Geometry check sheet. Reference: the model listing, model coordinates, mm. Round coordinates to 2 decimals unless told otherwise and drop trailing zeros. Write each loop counter-clockwise with the first axis right and the second up, starting at its lowest first coordinate (ties: lowest second). Pieces come first, ordered by that corner, then holes.
Item 1: Scan lines: probe 1 along Y at (x, z) = (589, 0); probe 2 along X at (y, z) = (-140, -45); probe 3 along Z at (x, y) = (953, 23). Record each from-to range of solid material in increasing order.
Item 2: Depth check by flat-ended pin: P1, Ø5, axis at x = 296, z = 9.5, coming from the -Y side; P2, Ø12, axis at x = 477, y = -91.5, coming from the -Z side; P3, Ø4, axis at x = 414, y = 117.5, coming from the +Z side. Enter the tip coordinate at first touch or a pass-through.
Item 3: Cross-section at C-C (x = 1178). Enter the section's corners in (y, z).
Item 4: Cross-section at A-A (y = 0). Enter the section's corners in (x, z).
from build123d import *

# Parameters (mm, degrees)
SKETCH1_R           = 158.75
SKETCH1_R_2         = 95.25
BOSS_EXTRUDE1_DEPTH = 1270
FILLET1_R           = 12.7
FILLET2_R           = 12.7


with BuildPart() as part:
    # Sketch1 → Boss-Extrude1 (new body)
    with BuildSketch(Plane(origin=(0, 0, 0), x_dir=(0, 0, -1), z_dir=(1, 0, 0))):
        Circle(SKETCH1_R)
        Circle(SKETCH1_R_2, mode=Mode.SUBTRACT)
    extrude(amount=BOSS_EXTRUDE1_DEPTH)

    # Fillet1
    fillet1_edges = [part.edges().sort_by_distance(p)[0] for p in [
        (1270, 0, 158.75),
        (1270, 0, 95.25),
    ]]
    fillet(fillet1_edges, radius=FILLET1_R)

    # Fillet2
    fillet2_edges = [part.edges().sort_by_distance(p)[0] for p in [
        (0, 0, 158.75),
        (0, 0, 95.25),
    ]]
    fillet(fillet2_edges, radius=FILLET2_R)


solid = part.part
Resolved:
1. probe 1: y = -158.75 to -95.25, 95.25 to 158.75
1. probe 2: x = 0.04 to 1269.96
1. probe 3: z = -157.08 to -92.43, 92.43 to 157.08
2. P1: stops at y = -158.6
2. P2: stops at z = -133.76
2. P3: stops at z = 108.91
3. outline: circle Ø317.5 at (0, 0); hole circle Ø190.5 at (0, 0)
4. outline: (0, -146.05) arc R12.7 ccw to (12.7, -158.75) - (1257.3, -158.75) arc R12.7 ccw to (1270, -146.05) - (1270, -107.95) arc R12.7 ccw to (1257.3, -95.25) - (12.7, -95.25) arc R12.7 ccw to (0, -107.95) - close; (0, 107.95) arc R12.7 ccw to (12.7, 95.25) - (1257.3, 95.25) arc R12.7 ccw to (1270, 107.95) - (1270, 146.05) arc R12.7 ccw to (1257.3, 158.75) - (12.7, 158.75) arc R12.7 ccw to (0, 146.05) - close
